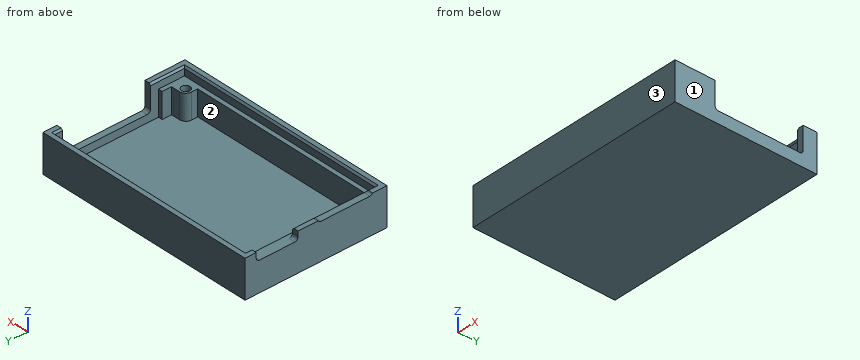
```python
from build123d import *

# Parameters (mm, degrees)
EXTRUDE_1_DEPTH     = 1
SKETCH_1_R          = 1
EXTRUDE_1_2_DEPTH   = 1
SKETCH_1_3_R        = 1.486
SKETCH_1_3_R_2      = 1
EXTRUDE_2_DEPTH     = 7
SKETCH_1_4_W        = 53.184
SKETCH_1_4_H        = 33.88
SKETCH_1_4_W_2      = 50.184
SKETCH_1_4_H_2      = 30.88
EXTRUDE_3_DEPTH     = 9
SKETCH_2_W          = 6.2
SKETCH_2_H          = 21
CUT_EXTRUDE_1_DEPTH = 62.545010001
SKETCH_3_W          = 2
SKETCH_3_H          = 10
CUT_EXTRUDE_2_DEPTH = 62.545010001
SKETCH_4_W          = 0.4
SKETCH_4_H          = 13
CUT_EXTRUDE_3_DEPTH = 62.545010001
FILLET_1_R          = 0.8
CHAMFER_1_SIZE      = 0.4


# Some blends are built 0.0001 mm under size
with BuildPart() as part:
    # Sketch 1 → Extrude 1 (new body)
    with BuildSketch(Plane.XY):
        with BuildLine():
            Line((48.984, 3.772), (48.984, 6))
            Line((48.984, 6), (49.984, 6))
            Line((49.984, 6), (49.984, 29.68))
            Line((49.984, 29.68), (0.8, 29.68))
            Line((0.8, 29.68), (0.8, 0.8))
            Line((0.8, 0.8), (45.377, 0.8))
            Line((45.377, 0.8), (45.377, 2.286))
            ThreePointArc((45.377, 2.286), (45.812239323, 3.336760677), (46.863, 3.772))
            Line((46.863, 3.772), (48.984, 3.772))
        make_face()
    extrude(amount=EXTRUDE_1_DEPTH)



with BuildPart() as body_2:
    # Sketch 1 → Extrude 1 2 (new body)
    with BuildSketch(Plane.XY):
        with Locations((46.863, 2.286)):
            Circle(SKETCH_1_R)
    extrude(amount=EXTRUDE_1_2_DEPTH)


with BuildPart() as part_1:
    add(part.part)

    add(body_2.part)  # Extrude 2 merges body 2
    # Sketch 1_3 → Extrude 2 (add)
    # profile 1 of 4: a face of its own
    with BuildSketch(Plane.XY):
        Polygon((0.8, 29.68), (48.984, 29.68), (49.984, 29.68), (49.984, 30.68), (-0.2, 30.68), (-0.2, -0.2), (49.984, -0.2), (49.984, 6), (48.984, 6), (48.984, 3.772), (48.984, 0.8), (46.863, 0.8), (45.377, 0.8), (0.8, 0.8), align=None)
    # profile 2 of 4: a face of its own
    with BuildSketch(Plane.XY):
        with BuildLine():
            Line((48.984, 0.8), (48.984, 3.772))
            Line((48.984, 3.772), (46.863, 3.772))
            ThreePointArc((46.863, 3.772), (47.913760677, 3.336760677), (48.349, 2.286))
            ThreePointArc((48.349, 2.286), (47.913760677, 1.235239323), (46.863, 0.8))
            Line((46.863, 0.8), (48.984, 0.8))
        make_face()
    # profile 3 of 4: a face of its own
    with BuildSketch(Plane.XY):
        with BuildLine():
            Line((45.377, 2.286), (45.377, 0.8))
            Line((45.377, 0.8), (46.863, 0.8))
            ThreePointArc((46.863, 0.8), (45.812239323, 1.235239323), (45.377, 2.286))
        make_face()
    # profile 4 of 4: a face of its own
    with BuildSketch(Plane.XY):
        with Locations((46.863, 2.286)):
            Circle(SKETCH_1_3_R)
        with Locations((46.863, 2.286)):
            Circle(SKETCH_1_3_R_2, mode=Mode.SUBTRACT)
    extrude(amount=EXTRUDE_2_DEPTH)

    # Sketch 1_4 → Extrude 3 (add)
    with BuildSketch(Plane.XY):
        with Locations((24.892, 15.24)):
            Rectangle(SKETCH_1_4_W, SKETCH_1_4_H)
        with Locations((24.892, 15.24)):
            Rectangle(SKETCH_1_4_W_2, SKETCH_1_4_H_2, mode=Mode.SUBTRACT)
    extrude(amount=EXTRUDE_3_DEPTH)

    # Sketch 2 → Cut-Extrude 1 (cut, through all)
    with BuildSketch(Plane.ZY.offset(-49.984)):
        with Locations((5.9, 18.374)):
            Rectangle(SKETCH_2_W, SKETCH_2_H)
    extrude(amount=-CUT_EXTRUDE_1_DEPTH, mode=Mode.SUBTRACT)

    # Sketch 3 → Cut-Extrude 2 (cut, through all)
    with BuildSketch(Plane(origin=(-0.2, 0, 0), x_dir=(0, 0, -1), z_dir=(1, 0, 0))):
        with Locations((-8, 24.5)):
            Rectangle(SKETCH_3_W, SKETCH_3_H)
    extrude(amount=-CUT_EXTRUDE_2_DEPTH, mode=Mode.SUBTRACT)

    # Sketch 4 → Cut-Extrude 3 (cut, through all)
    with BuildSketch(Plane(origin=(-0.2, 0, 0), x_dir=(0, 0, -1), z_dir=(1, 0, 0))):
        with Locations((-8.8, 8.25)):
            Rectangle(SKETCH_4_W, SKETCH_4_H)
    extrude(amount=-CUT_EXTRUDE_3_DEPTH, mode=Mode.SUBTRACT)

    # Fillet 1
    # the kernel refuses this fillet: 0.8 mm, written as the material it adds along each edge
    with BuildSketch(Plane(origin=(49.984, 7.874, 2.8), x_dir=(0, 1, 0), z_dir=(1, 0, 0)), Plane(origin=(49.984, 28.874, 2.8), x_dir=(0, 0, 1), z_dir=(1, 0, 0)), Plane(origin=(-0.2, 19.5, 7), x_dir=(0, 0, 1), z_dir=(-1, 0, 0)), Plane(origin=(-0.2, 29.5, 7), x_dir=(0, -1, 0), z_dir=(-1, 0, 0))) as fillet_1_piece_1:
        with BuildLine():
            CenterArc((FILLET_1_R, FILLET_1_R), FILLET_1_R, 180, 90)
            Line((0, FILLET_1_R), (-FILLET_1_R * 0.02, FILLET_1_R))
            Line((-FILLET_1_R * 0.02, FILLET_1_R), (-FILLET_1_R * 0.02, -FILLET_1_R * 0.02))
            Line((-FILLET_1_R * 0.02, -FILLET_1_R * 0.02), (FILLET_1_R, -FILLET_1_R * 0.02))
            Line((FILLET_1_R, -FILLET_1_R * 0.02), (FILLET_1_R, 0))
        make_face()
    extrude(amount=1.5)
    with BuildSketch(Plane(origin=(-0.2, 1.75, 8.6), x_dir=(0, 0, 1), z_dir=(-1, 0, 0))) as fillet_1_piece_2:
        with BuildLine():
            CenterArc((0.8, 0.692820323), FILLET_1_R, 180, 60)
            Line((0, 0.692820323), (-0.016, 0.692820323))
            Line((-0.016, 0.692820323), (-0.016, 0))
            Line((-0.016, 0), (0, -0.016))
            ThreePointArc((0, -0.016), (0.2, -0.016), (0.392, -0.013856406))
            Line((0.392, -0.013856406), (0.4, 0))
        make_face()
    extrude(amount=1.5)
    with BuildSketch(Plane(origin=(-0.2, 14.75, 8.6), x_dir=(0, -1, 0), z_dir=(-1, 0, 0))) as fillet_1_piece_3:
        with BuildLine():
            CenterArc((0.692820323, 0.8), FILLET_1_R, 210, 60)
            Line((0, 0.4), (-0.013856406, 0.392))
            ThreePointArc((-0.013856406, 0.392), (-0.016, 0.2), (-0.016, 0))
            Line((-0.016, 0), (0, -0.016))
            Line((0, -0.016), (0.692820323, -0.016))
            Line((0.692820323, -0.016), (0.692820323, 0))
        make_face()
    extrude(amount=1.5)

    # Chamfer 1
    chamfer_1_edges = [part_1.edges().sort_by_distance(p)[0] for p in [
        (-0.2, 17.125, 9),
        (-0.2, 0.775, 9),
        (24.892, -0.2, 9),
        (49.984, 3.837, 9),
        (49.984, 29.777, 9),
        (24.892, 30.68, 9),
        (-0.2, 30.09, 9),
    ]]
    chamfer(chamfer_1_edges, length=CHAMFER_1_SIZE - 0.0001)  # a hair under: the kernel refuses the full size


solid = part_1.part
```
Model file for the job. Use its own axes, mm. Face numbers are marked on the shaded views. Round coordinates to 2 decimals unless told otherwise and drop trailing zeros. Loops run counter-clockwise (first coordinate to the right, second up) from the corner with the lowest first, then second, coordinate; pieces in that order, holes last. Notation, with made-up numbers: M 19.5,48 L 71.5,48 A10 cw 71.5,62 Z; hole C 72.5,41 d1. An arc over 180 degrees is marked long. Put each result on its own line as item: value. Start each with the question number.
Item 1: Drill centre lines: line 1 along Y through (x, z) = (45, 3.5); line 2 along X through (y, z) = (4, 6); line 3 along X through (y, z) = (21, 2.25). Where is each one in solid material? Low to high.
Item 2: Drop flat-ended pins along their axis: P1, Ø8, axis at x = 11.5, y = 11.5, coming from the +Z side; P2, Ø0.8, axis at x = -1, y = 10, coming from the +Z side; P3, Ø5, axis at x = 37.5, y = 15, coming from the -Z side. Give the stop position or say it passes through.
Item 3: Cut at A-A (x = 17.5). List the corners of the cut face in (y, z), then the cut area to 3 significant figures.
Item 4: Cut at B-B (y = 17.5). List the corners of the cut face in (x, z).
Item 5: Cut at C-C (y = 21.5). List the corners of the cut face in (x, z).
Item 6: Mould opens along Y. For the marked faces 1, 2 and 3 say: released by +Y, released by -Y, zero draft, split by the parting line, or undercut.
Answer block:
1. line 1: -1.7 to 0.8, 29.68 to 32.18
1. line 2: -1.7 to 0.8, 48.98 to 51.48
1. line 3: -1.7 to 0.8, 49.98 to 51.48
2. P1: z = 1
2. P2: z = 8.6
2. P3: z = 0
3. outline: M -1.7,0 L 32.18,0 L 32.18,9 L 31.08,9 L 30.68,8.6 L 30.68,7 L 29.68,7 L 29.68,1 L 0.8,1 L 0.8,7 L -0.2,7 L -0.2,8.6 L -0.6,9 L -1.7,9 Z
3. area: 69.7 mm2
4. outline: M -1.7,0 L 51.48,0 L 51.48,2.8 L 49.98,2.8 L 49.98,1 L 0.8,1 L 0.8,7 L -0.2,7 L -0.2,8.6 L -0.6,9 L -1.7,9 Z
5. outline: M -1.7,0 L 51.48,0 L 51.48,2.8 L 49.98,2.8 L 49.98,1 L 0.8,1 L 0.8,7 L -1.7,7 Z
6. face 1: zero draft
6. face 2: undercut
6. face 3: released by -Y
